Can you work these out from the model? Positions are in its coordinate system, mm. A direction names the side the tool comes from. Coordinates: 2 decimals unless noted, no trailing zeros. Loops run counter-clockwise (first coordinate to the right, second up) from the corner with the lowest first, then second, coordinate; pieces in that order, holes last.
```python
from build123d import *

# Parameters (mm, degrees)
SKETCH_1_R          = 25
EXTRUDE_1_DEPTH     = 3
SKETCH_2_R          = 1.6
SKETCH_2_R_2        = 1.5
CUT_EXTRUDE_1_DEPTH = 3
CUT_EXTRUDE_START   = -3
SKETCH_3_R          = 25
CUT_EXTRUDE_2_DEPTH = 3
FILLET_1_R          = 0.5
SKETCH_4_W          = 17.9
SKETCH_4_H          = 6.05
CUT_EXTRUDE_3_DEPTH = 10
FILLET_3_R          = 2.03
CUT_EXTRUDE_START_2 = -2.3
CUT_EXTRUDE_5_DEPTH = 2.3
FILLET_4_R          = 2
CHAMFER_1_SIZE      = 0.5
FILLET_7_R          = 1
CHAMFER_3_SIZE      = 0.5


with BuildPart() as part:
    # 草图1 → 凸台-拉伸1 (new body)
    with BuildSketch(Plane(origin=(0, 0, 0), x_dir=(1, 0, 0), z_dir=(0, 1, 0))):
        with Locations(Location((0, 0, 0), (0, 0, 270))):
            Circle(SKETCH_1_R)
    extrude(amount=EXTRUDE_1_DEPTH)

    # 草图2 → 切除-拉伸1 (cut)
    with BuildSketch(Plane(origin=(0, 3, 0), x_dir=(1, 0, 0), z_dir=(0, 1, 0))):
        with Locations(Location((10.392304845, -6, 0), (0, 0, 270))):
            Circle(SKETCH_2_R)
        with Locations(Location((-10.392304845, -6, 0), (0, 0, 270))):
            Circle(SKETCH_2_R)
        with Locations(Location((0, 12, 0), (0, 0, 270))):
            Circle(SKETCH_2_R)
        with Locations(Location((0, -12, 0), (0, 0, 270))):
            Circle(SKETCH_2_R_2)
        with Locations(Location((-10.392304845, 6, 0), (0, 0, 270))):
            Circle(SKETCH_2_R_2)
        with Locations(Location((10.392304845, 6, 0), (0, 0, 270))):
            Circle(SKETCH_2_R_2)
    extrude(amount=-CUT_EXTRUDE_1_DEPTH, mode=Mode.SUBTRACT)

    # 草图3 → 切除-拉伸2 (cut)
    with BuildSketch(Plane(origin=(0, 3, 0), x_dir=(1, 0, 0), z_dir=(0, 1, 0)).offset(CUT_EXTRUDE_START)):
        Circle(SKETCH_3_R)
        with BuildLine():
            Line((-6.211657082, 23.182219831), (-5.176380902, 19.318516526))
            ThreePointArc((-5.176380902, 19.318516526), (0, -20), (5.176380902, 19.318516526))
            Line((5.176380902, 19.318516526), (6.211657082, 23.182219831))
            ThreePointArc((6.211657082, 23.182219831), (0, 24), (-6.211657082, 23.182219831))
        make_face(mode=Mode.SUBTRACT)
    extrude(amount=CUT_EXTRUDE_2_DEPTH, mode=Mode.SUBTRACT)

    # 圆角1
    fillet_1_edges = [part.edges().sort_by_distance(p)[0] for p in [
        (5.176380902, 1.5, -19.318516526),
        (-5.176380902, 1.5, -19.318516526),
    ]]
    fillet(fillet_1_edges, radius=FILLET_1_R)

    # 草图4 → 切除-拉伸3 (cut)
    with BuildSketch(Plane(origin=(0, 3, 0), x_dir=(1, 0, 0), z_dir=(0, 1, 0))):
        Rectangle(SKETCH_4_W, SKETCH_4_H)
    extrude(amount=-CUT_EXTRUDE_3_DEPTH, mode=Mode.SUBTRACT)

    # 圆角3
    fillet_3_edges = [part.edges().sort_by_distance(p)[0] for p in [
        (8.95, 1.5, -3.025),
        (8.95, 1.5, 3.025),
        (-8.95, 1.5, 3.025),
        (-8.95, 1.5, -3.025),
    ]]
    fillet(fillet_3_edges, radius=FILLET_3_R)

    # 草图5 → 切除-拉伸5 (cut)
    with BuildSketch(Plane(origin=(0, 3, 0), x_dir=(1, 0, 0), z_dir=(0, 1, 0)).offset(CUT_EXTRUDE_START_2)):
        with BuildLine():
            Line((-3.5, 23.743420141), (-3.5, 17))
            Line((-3.5, 17), (3.5, 17))
            Line((3.5, 17), (3.5, 23.743420141))
            ThreePointArc((3.5, 23.743420141), (0, 24), (-3.5, 23.743420141))
        make_face()
    extrude(amount=CUT_EXTRUDE_5_DEPTH, mode=Mode.SUBTRACT)

    # 圆角4
    fillet_4_edges = [part.edges().sort_by_distance(p)[0] for p in [
        (-3.5, 1.85, -17),
        (3.5, 1.85, -17),
    ]]
    fillet(fillet_4_edges, radius=FILLET_4_R)

    # 倒角1
    chamfer_1_edges = [part.edges().sort_by_distance(p)[0] for p in [
        (-8.355426766, 0, 2.430426766),
        (-8.355426766, 3, -2.430426766),
        (-8.355426766, 0, -2.430426766),
        (0, 0, 10.5),
        (0, 3, 10.5),
        (-10.392304845, 0, 4.4),
        (-10.392304845, 3, 4.4),
        (10.392304845, 0, -7.5),
        (10.392304845, 3, -7.5),
        (-10.392304845, 0, -7.5),
        (-10.392304845, 3, -7.5),
        (10.392304845, 0, 4.4),
        (10.392304845, 3, 4.4),
        (0, 0, -13.6),
        (0, 3, -13.6),
        (0, 0, -24),
        (-5.757934554, 0, -21.488904301),
        (-5.757934554, 3, -21.488904301),
        (0, 3, 20),
        (0, 0, 20),
        (5.757934554, 3, -21.488904301),
        (5.757934554, 0, -21.488904301),
        (5.351145434, 3, -19.421478878),
        (5.351145434, 0, -19.421478878),
        (-5.351145434, 3, -19.421478878),
        (-5.351145434, 0, -19.421478878),
        (8.95, 3, 0),
        (8.95, 0, 0),
        (0, 3, 3.025),
        (0, 0, 3.025),
        (0, 3, -3.025),
        (0, 0, -3.025),
        (-8.95, 3, 0),
        (-8.95, 0, 0),
        (8.355426766, 3, 2.430426766),
        (8.355426766, 0, 2.430426766),
        (8.355426766, 3, -2.430426766),
        (8.355426766, 0, -2.430426766),
        (-8.355426766, 3, 2.430426766),
    ]]
    chamfer(chamfer_1_edges, length=CHAMFER_1_SIZE)

    # 圆角7
    fillet_7_edges = [part.edges().sort_by_distance(p)[0] for p in [
        (-3.5, 1.85, -23.743420141),
        (3.5, 1.85, -23.743420141),
        (-6.211657082, 1.5, -23.182219831),
        (6.211657082, 1.5, -23.182219831),
    ]]
    fillet(fillet_7_edges, radius=FILLET_7_R)

    # 倒角3
    chamfer_3_edges = [part.edges().sort_by_distance(p)[0] for p in [
        (4.947039166, 3, -23.484607799),
        (3.865828168, 3, -23.328679278),
        (3.5, 3, -20.777743569),
        (2.914213562, 3, -17.585786438),
        (0, 3, -17),
        (-2.914213562, 3, -17.585786438),
        (-3.5, 3, -20.777743569),
        (-4.947039166, 3, -23.484607799),
        (-3.865828168, 3, -23.328679278),
        (5.46233374, 3, -23.33079751),
        (-5.46233374, 3, -23.33079751),
    ]]
    chamfer(chamfer_3_edges, length=CHAMFER_3_SIZE - 0.0001)  # a hair under: the kernel refuses the full size


solid = part.part
```
Item 1: We'd pull the mould along X, two halves only. Please class faces 1 (the face through (-11.305, 1.514, -7.19)), 2 (the face through (5.47, 0.25, -21.39)), 3 (the face through (0, 0, -7)): +X half, -X half, draft (parallel to the pull), parting line (faces both ways), or undercut.
Results are:
face 1: undercut
face 2: +X half
face 3: draft
Item 2: Suppose I cut it at A-A, the plane z = 0. Please give me the cut outline in (x, y).
Results are:
outline: (-20, 0.5) - (-19.5, 0) - (-9.45, 0) - (-8.95, 0.5) - (-8.95, 2.5) - (-9.45, 3) - (-19.5, 3) - (-20, 2.5) - close; (8.95, 0.5) - (9.45, 0) - (19.5, 0) - (20, 0.5) - (20, 2.5) - (19.5, 3) - (9.45, 3) - (8.95, 2.5) - close
Item 3: I need wall thicknesses on line 1 along X through (y, z) = (1.3, 6); line 2 along X through (y, z) = (1.7, -5); line 3 along Z through (x, y) = (8.5, 1.4). Which ranges of each line are inside material? Lowest first, please.
Results are:
line 1: x = -19.08 to -11.99, -8.79 to 8.79, 11.99 to 19.08
line 2: x = -19.36 to -11.51, -9.27 to 9.27, 11.51 to 19.36
line 3: z = -18.1 to -2.27, 2.27 to 18.1
Item 4: Suppose I cut it at B-B, the plane x = 0. Count the separate pieces of the cut face and the enclosed holes in it, plus the area to 4 significant figures.
Results are:
separate pieces: 4
enclosed holes: 0
area: 77.15 mm2
Item 5: I'm going to push flat-ended pins straight in: P1, Ø1.4, axis at y = 1.5, z = -21, coming from the +X side; P2, Ø1.5, axis at x = 14.5, y = 2, coming from the -Z side; P3, Ø1, axis at x = 15, y = 2.5, coming from the -Z side (3 decimals). Where does each tip first touch, or does it pass through?
Results are:
P1: stops at x = 5.81
P2: stops at z = -14.52
P3: stops at z = -13.775
Item 6: On a 3-axis mill with a long thin cutter (end or side, diameter ignored), from which of +Z, -Z, +X, -X, +Y, -Y can I reach the whole of each face in a straight line? I mean faces 4 (the face through (0, 3, -7)), 5 (the face through (-8.439, 0.358, 2.548)), 6 (the face through (3.88, 1.61, -23.34)), 7 (the face through (8.47, 2.64, -2.51)), 8 (the face through (0, 2, -3.025)). Say none if no direction works.
Results are:
face 4: +Z, -Z, +X, -X, +Y
face 5: -Y
face 6: -Z, +Y
face 7: +Y
face 8: +Y, -Y
